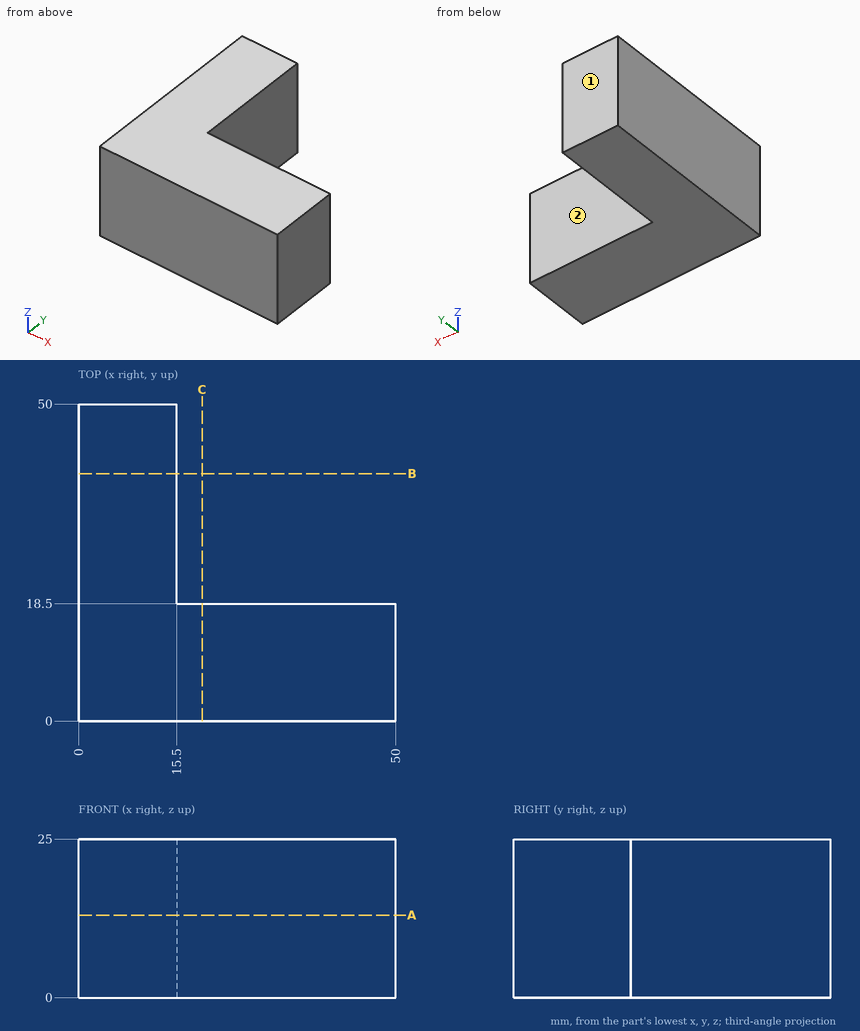
Geometry check sheet. Reference: drawing and pictorial views, mm from the part's lowest x, y, z. A direction names the side the tool comes from. Round coordinates to 2 decimals unless told otherwise and drop trailing zeros. Write each loop counter-clockwise with the first axis right and the second up, starting at its lowest first coordinate (ties: lowest second). Pieces come first, ordered by that corner, then holes.
(1) Section check A-A (z = 13). Enter the section's corners in (x, y), plus the area to 3 significant figures.
Returned:
outline: (0, 0) - (50, 0) - (50, 18.5) - (15.5, 18.5) - (15.5, 50) - (0, 50) - close
area: 1,410 mm2
(2) Section check C-C (x = 19.5). Enter the section's corners in (y, z).
Returned:
outline: (0, 0) - (18.5, 0) - (18.5, 25) - (0, 25) - close
(3) Section check B-B (y = 39). Enter the section's corners in (x, z).
Returned:
outline: (0, 0) - (15.5, 0) - (15.5, 25) - (0, 25) - close
(4) Depth check by flat-ended pin: pin 1 Ø1 at (x, y) = (21, 20.5) entering from +Z; pin 2 Ø10 at (x, z) = (27, 16) entering from +Y; pin 3 Ø6 at (y, z) = (39, 11) entering from +X. Enter the tip coordinate at first touch or a pass-through.
Returned:
pin 1: passes through
pin 2: stops at y = 18.5
pin 3: stops at x = 15.5
(5) Material ranges on line 1 (X direction, y = 22.5, z = 15.5); line 2 (Y direction, x = 18.5, z = 14.25), recorded low to high.
Returned:
line 1: x = 0 to 15.5
line 2: y = 0 to 18.5
(6) Access from +Z, -Z, +X, -X, +Y, -Y to the whole of each face (thin tool, end or side, straight path). Record for the marked faces 1 and 2.
Returned:
face 1: +Z, -Z, +X, -X, +Y
face 2: +Z, -Z, +X, +Y
